```python
from build123d import *

# Parameters (mm, degrees)
SKETCH1_W           = 10
SKETCH1_H           = 12
SKETCH1_R           = 1.5
BOSS_EXTRUDE1_DEPTH = 2
SKETCH2_W           = 10
SKETCH2_H           = 13
BOSS_EXTRUDE2_DEPTH = 2
SKETCH3_W           = 10
SKETCH3_H           = 50
BOSS_EXTRUDE3_DEPTH = 2
SKETCH4_W           = 10
SKETCH4_H           = 26
SKETCH4_R           = 3
BOSS_EXTRUDE4_DEPTH = 2
FILLET1_R           = 1
FILLET2_R           = 1
FILLET3_R           = 1
FILLET4_R           = 1
FILLET5_R           = 1
FILLET6_R           = 1


with BuildPart() as part:
    # Sketch1 → Boss-Extrude1 (new body)
    with BuildSketch(Plane(origin=(0, 0, 0), x_dir=(1, 0, 0), z_dir=(0, 1, 0))):
        with Locations((-0.086956522, 1.043478261)):
            Rectangle(SKETCH1_W, SKETCH1_H)
        with Locations(Location((-0.086956522, -1.456521739, 0), (0, 0, 270))):
            Circle(SKETCH1_R, mode=Mode.SUBTRACT)
        with Locations(Location((-0.086956522, 3.543478261, 0), (0, 0, 270))):
            Circle(SKETCH1_R, mode=Mode.SUBTRACT)
    extrude(amount=BOSS_EXTRUDE1_DEPTH)

    # Sketch2 → Boss-Extrude2 (add)
    with BuildSketch(Plane.XY.offset(4.956521739)):
        with Locations((-0.086956522, 6.5)):
            Rectangle(SKETCH2_W, SKETCH2_H)
    extrude(amount=BOSS_EXTRUDE2_DEPTH)

    # Sketch3 → Boss-Extrude3 (add)
    with BuildSketch(Plane(origin=(0, 13, 0), x_dir=(1, 0, 0), z_dir=(0, 1, 0))):
        with Locations((-0.086956522, -29.956521739)):
            Rectangle(SKETCH3_W, SKETCH3_H)
    extrude(amount=BOSS_EXTRUDE3_DEPTH)

    # Sketch4 → Boss-Extrude4 (add)
    with BuildSketch(Plane.XY.offset(54.956521739)):
        with Locations((-0.086956522, 2)):
            Rectangle(SKETCH4_W, SKETCH4_H)
        with Locations((-0.086956522, -6.5)):
            Circle(SKETCH4_R, mode=Mode.SUBTRACT)
    extrude(amount=BOSS_EXTRUDE4_DEPTH)

    # Fillet1
    fillet1_edges = [part.edges().sort_by_distance(p)[0] for p in [
        (-0.086956522, 15, 56.956521739),
    ]]
    fillet(fillet1_edges, radius=FILLET1_R)

    # Fillet2
    fillet2_edges = [part.edges().sort_by_distance(p)[0] for p in [
        (-0.086956522, 13, 54.956521739),
    ]]
    fillet(fillet2_edges, radius=FILLET2_R)

    # Fillet3
    fillet3_edges = [part.edges().sort_by_distance(p)[0] for p in [
        (-0.086956522, 15, 4.956521739),
    ]]
    fillet(fillet3_edges, radius=FILLET3_R)

    # Fillet4
    fillet4_edges = [part.edges().sort_by_distance(p)[0] for p in [
        (-0.086956522, 13, 6.956521739),
    ]]
    fillet(fillet4_edges, radius=FILLET4_R)

    # Fillet5
    fillet5_edges = [part.edges().sort_by_distance(p)[0] for p in [
        (-0.086956522, 0, 6.956521739),
    ]]
    fillet(fillet5_edges, radius=FILLET5_R)

    # Fillet6
    fillet6_edges = [part.edges().sort_by_distance(p)[0] for p in [
        (-0.086956522, 2, 4.956521739),
    ]]
    fillet(fillet6_edges, radius=FILLET6_R)


solid = part.part
```
Model file for the job. Use its own axes, mm. A direction names the side the tool comes from. Give positions to 0.01 mm unless a question says otherwise; leave off trailing zeros. Order: outer loops, then holes, each group sorted by start corner. A loop starts at its lowest first (then second) coordinate and runs counter-clockwise, first axis right, second up.
1) Saw through at C-C, the plane y = -6.5. Write the cut outline in (x, z).
2) 3-axis set-ups, long thin cutter, end or side, ignore diameter. For faces 1 (the flat face through (-0.2, 2, -1.6)), 2 (the flat face through (0, 0, -1)), 3 (the flat face through (0, 13, 31)): which of +Z, -Z, +X, -X, +Y, -Y reach the whole face in a straight line?
3) Pin check, flat tips, straight feed: pin 1 (12 mm diameter, centred on y = 5, z = 23.5, fed in from -X); pin 2 (3 mm diameter, centred on x = 0, y = -2, fed in from -Z); pin 3 (5 mm diameter, centred on x = -1, z = 26.5, fed in from -Y); pin 4 (3 mm diameter, centred on x = -2, y = 6.5, fed in from -Z). Stop position of each tip, or through.
4) Mould opens along X. For faces 4 (the cylindrical face through (1.526, -3.97, 55.943)), 5 (the flat face through (-5.087, 13.5, 29.5)), 6 (the cylindrical face through (-1.55, 0.99, -3.87)), 7 (the flat face through (0, -11, 56)) say: +X half, -X half, draft (parallel to the pull), parting line (faces both ways), or undercut.
5) Saw through at A-A, the plane y = 4.25. Write the cut outline in (x, z), then the cut area to 3 significant figures.
6) Saw through at B-B, the plane x = 2.25. Write the cut outline in (y, z).
7) Saw through at D-D, the plane z = 31.5. Write the cut outline in (x, y), then the cut area to 3 significant figures.
8) Wall check: probe 1 along Z at (x, y) = (-4, 3.5); probe 2 along Y at (x, z) = (-2.5, 23); probe 3 along Z at (x, y) = (-4.5, -8). Give the ranges that are in metal, low to high.
Computed:
1. outline: (-5.09, 54.96) - (-3.09, 54.96) - (-3.09, 56.96) - (-5.09, 56.96) - close; (2.91, 54.96) - (4.91, 54.96) - (4.91, 56.96) - (2.91, 56.96) - close
2. face 1: -Z, +X, -X, +Y
2. face 2: -Z, +X, -X, -Y
2. face 3: +X, -X, -Y
3. pin 1: passes through
3. pin 2: stops at z = 54.96
3. pin 3: stops at y = 13
3. pin 4: stops at z = 4.96
4. face 4: undercut
4. face 5: -X half
4. face 6: undercut
4. face 7: draft
5. outline: (-5.09, 4.96) - (4.91, 4.96) - (4.91, 6.96) - (-5.09, 6.96) - close; (-5.09, 54.96) - (4.91, 54.96) - (4.91, 56.96) - (-5.09, 56.96) - close
5. area: 40.0 mm2
6. outline: (-11, 54.96) - (-8.38, 54.96) - (-8.38, 56.96) - (-11, 56.96) - close; (-4.62, 54.96) - (12, 54.96) arc R1 cw to (13, 53.96) - (13, 7.96) arc R1 cw to (12, 6.96) - (1, 6.96) arc R1 ccw to (0, 5.96) - (0, -7.04) - (2, -7.04) - (2, 3.96) arc R1 cw to (3, 4.96) - (14, 4.96) arc R1 ccw to (15, 5.96) - (15, 55.96) arc R1 ccw to (14, 56.96) - (-4.62, 56.96) - close
7. outline: (-5.09, 13) - (4.91, 13) - (4.91, 15) - (-5.09, 15) - close
7. area: 20.0 mm2
8. probe 1: z = 4.96 to 6.96, 54.96 to 56.96
8. probe 2: y = 13 to 15
8. probe 3: z = 54.96 to 56.96
